Model file for the job. Use its own axes, mm. Face numbers are marked on the shaded views. A direction names the side the tool comes from. Give positions to 0.01 mm unless a question says otherwise; leave off trailing zeros. Loops run counter-clockwise (first coordinate to the right, second up) from the corner with the lowest first, then second, coordinate; pieces in that order, holes last. Notation, with made-up numbers: (28.25, -32) - (35.25, -32) arc R8 cw to (35.25, -22) - close; hole circle Ø6 at (72, -5.5). An arc over 180 degrees is marked (long way). Use a Markdown table: item, result.
from build123d import *

# Parameters (mm, degrees)
SKETCH_1_W      = 43
SKETCH_1_H      = 25
EXTRUDE_1_DEPTH = 1
SKETCH_3_W      = 34
SKETCH_3_H      = 22
EXTRUDE_2_DEPTH = 4
SKETCH_4_W      = 6.5
SKETCH_4_H      = 6.5
EXTRUDE_3_DEPTH = 1.5
SKETCH_5_R      = 3
EXTRUDE_4_DEPTH = 12.5
SKETCH_6_R      = 4.75
EXTRUDE_5_DEPTH = 3


with BuildPart() as part:
    # 草图1 → 凸台-拉伸1 (new body)
    with BuildSketch(Plane.XY):
        Rectangle(SKETCH_1_W, SKETCH_1_H)
    extrude(amount=-EXTRUDE_1_DEPTH)

    # 草图3 → 凸台-拉伸2 (add)
    with BuildSketch(Plane.XY):
        with Locations((-1.5, 0)):
            Rectangle(SKETCH_3_W, SKETCH_3_H)
    extrude(amount=-EXTRUDE_2_DEPTH)

    # 草图4 → 凸台-拉伸3 (add)
    with BuildSketch(Plane(origin=(21.5, 0, 0), x_dir=(0, 0, -1), z_dir=(1, 0, 0))):
        with Locations((1.75, 7.5)):
            Rectangle(SKETCH_4_W, SKETCH_4_H)
    extrude(amount=EXTRUDE_3_DEPTH)

    # 草图5 → 凸台-拉伸4 (add)
    with BuildSketch(Plane.ZY.offset(-21.5)):
        with Locations((-1.75, 7.5)):
            Circle(SKETCH_5_R)
    extrude(amount=-EXTRUDE_4_DEPTH)

    # 草图6 → 凸台-拉伸5 (add)
    with BuildSketch(Plane(origin=(23, 0, 0), x_dir=(0, 0, -1), z_dir=(1, 0, 0))):
        with Locations((1.75, 7.5)):
            Circle(SKETCH_6_R)
    extrude(amount=EXTRUDE_5_DEPTH)


solid = part.part
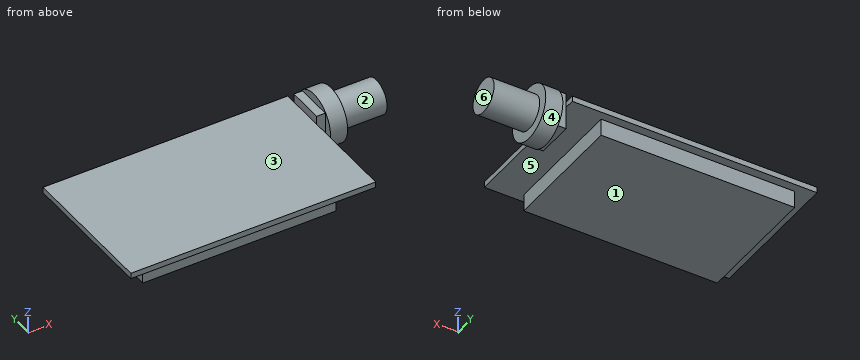
(1) Pin check, flat tips, straight feed: P1, Ø2, axis at x = 23.5, y = -0.5, coming from the +Z side; P2, Ø3, axis at x = 21, y = -9, coming from the +Z side; P3, Ø7.5, axis at x = 2, y = -0.5, coming from the -Z side; P4, Ø3, axis at y = 6, z = -3.5, coming from the -X side. Stop position of each tip, or through.
Computed:
| item | result |
|---|---|
| P1 | through |
| P2 | z = 0 |
| P3 | z = -4 |
| P4 | x = -18.5 |
(2) Drill centre lines: probe 1 along Z at (x, y) = (-6, -10.5); probe 2 along Y at (x, z) = (2, -2.5); probe 3 along X at (y, z) = (8.25, -4.5). Where is each one in solid material? Low to high. Write a range as [from, to].
Computed:
| item | result |
|---|---|
| probe 1 | [-4, 0] |
| probe 2 | [-11, 11] |
| probe 3 | [21.5, 34] |
(3) Slice it at C-C, the plane y = 2.25. Write the cut outline in (x, z), plus the area to 3 significant figures.
Computed:
| item | result |
|---|---|
| outline | (-21.5, -1) - (-18.5, -1) - (-18.5, -4) - (15.5, -4) - (15.5, -1) - (21.5, -1) - (21.5, 0) - (-21.5, 0) - close |
| area | 145 mm² |
(4) Mould opens along X. For the marked faces 4, 5 and 6 say: pulls with the +X half, pulls with the -X half, needs draft (parallel to the pull), parting line crosses it, or undercut.
Computed:
| item | result |
|---|---|
| face 4 | needs draft |
| face 5 | undercut |
| face 6 | pulls with the +X half |
(5) Slice it at D-D, the plane z = 0.75. Write the cut outline in (x, y), plus the area to 3 significant figures.
Computed:
| item | result |
|---|---|
| outline | (21.5, 4.25) - (23, 4.25) - (23, 3.46) - (26, 3.46) - (26, 5.84) - (34, 5.84) - (34, 9.16) - (26, 9.16) - (26, 11.54) - (23, 11.54) - (23, 10.75) - (21.5, 10.75) - close |
| area | 60.5 mm² |
(6) Slice it at B-B, the plane x = -14. Write the cut outline in (y, z).
Computed:
| item | result |
|---|---|
| outline | (-12.5, -1) - (-11, -1) - (-11, -4) - (11, -4) - (11, -1) - (12.5, -1) - (12.5, 0) - (-12.5, 0) - close |
(7) 3-axis set-ups, long thin cutter, end or side, ignore diameter. For the marked faces 1, 2 and 3: which of +Z, -Z, +X, -X, +Y, -Y reach the whole face in a straight line?
Computed:
| item | result |
|---|---|
| face 1 | -Z, -X, +Y, -Y |
| face 2 | +X |
| face 3 | +Z, -X, +Y, -Y |
(8) Slice it at A-A, the plane z = -1.75. Write the cut outline in (x, y).
Computed:
| item | result |
|---|---|
| outline | (-18.5, -11) - (15.5, -11) - (15.5, 11) - (-18.5, 11) - close; (21.5, 4.25) - (23, 4.25) - (23, 2.75) - (26, 2.75) - (26, 4.5) - (34, 4.5) - (34, 10.5) - (26, 10.5) - (26, 12.25) - (23, 12.25) - (23, 10.75) - (21.5, 10.75) - close |
